```python
from build123d import *

# Parameters (mm, degrees)
F0_W          = 18
F0_H          = 18
F0_W_2        = 10
F0_H_2        = 10
F1_DEPTH      = 4
F2_DEPTH      = 12
F2_TAPER      = 3
F3_SIZE       = 2
F4_R          = 2
F5_W          = 5
F5_H          = 5
F6_DEPTH      = 5
F6_TAPER      = 3
F7_W          = 6
F7_H          = 3
F8_DEPTH      = 25
F8_DEPTH_BACK = 25


with BuildPart() as f1:
    # F0 (on Top) → F1 (new body)
    with BuildSketch(Plane.XY):
        Rectangle(F0_W, F0_H)
        Rectangle(F0_W_2, F0_H_2, mode=Mode.SUBTRACT)
        Rectangle(F0_W_2, F0_H_2)
    extrude(amount=F1_DEPTH)

    # F0 (on Top) → F2 (join)
    with BuildSketch(Plane.XY):
        Rectangle(F0_W_2, F0_H_2)
    extrude(amount=F2_DEPTH, taper=F2_TAPER)

    # F3
    f3_edges = [f1.edges().sort_by_distance(p)[0] for p in [
        (-9, 0, 4),
        (0, -9, 4),
        (9, 0, 4),
        (0, 9, 4),
    ]]
    chamfer(f3_edges, length=F3_SIZE)

    # F4
    f4_edges = [f1.edges().sort_by_distance(p)[0] for p in [
        (0, -4.790369, 4),
        (-4.790369, 0, 4),
        (4.790369, 0, 4),
        (0, 4.790369, 4),
    ]]
    fillet(f4_edges, radius=F4_R)

    # F5 (on face) → F6 (cut)
    with BuildSketch(Plane.XY.offset(12)):
        Rectangle(F5_W, F5_H)
    extrude(amount=-F6_DEPTH, taper=F6_TAPER, mode=Mode.SUBTRACT)

    # F7 (on Front) → F8 (cut, two sides)
    with BuildSketch(Plane.XZ) as f8_sk:
        with Locations((0, 9)):
            Rectangle(F7_W, F7_H)
    extrude(amount=F8_DEPTH, mode=Mode.SUBTRACT)
    extrude(f8_sk.sketch, amount=-F8_DEPTH_BACK, mode=Mode.SUBTRACT)


solid = f1.part
```
Build history of the part. All positions in model axes, mm. A direction names the side the tool comes from. Round coordinates to 2 decimals unless told otherwise and drop trailing zeros. Loops run counter-clockwise (first coordinate to the right, second up) from the corner with the lowest first, then second, coordinate; pieces in that order, holes last. Notation, with made-up numbers: M -14,67.25 L 17,67.25 A20 cw 17,84.25 Z; hole C 31.5,67.5 d2. An arc over 180 degrees is marked long. Answer as CSV lines item,"result".
1. 3-axis set-ups, long thin cutter, end or side, ignore diameter. For faces 5 (the flat face through (0, 0, 7)), 6 (the flat face through (2.6, 0.1, 7.5)), 7 (the flat face through (0, 0, 0)): which of +Z, -Z, +X, -X, +Y, -Y reach the whole face in a straight line?
Resolved:
face 5,"+Z"
face 6,"+Y, -Y"
face 7,"-Z, +X, -X, +Y, -Y"
2. Two-plate mould, pull along Z, no slides. Class faces 1 (the flat face through (-9, 0, 1)), 2 (the flat face through (0, -8, 3)), 3 (the flat face through (3, 0, 9)), 4 (the flat face through (-3, 0, 9)): released by +Z, released by -Z, zero draft, split by the parting line, or undercut.
Resolved:
face 1,"zero draft"
face 2,"released by +Z"
face 3,"undercut"
face 4,"undercut"
3. Wall check: probe 1 along Z at (x, y) = (2.5, -3); probe 2 along X at (y, z) = (-2.25, 9); probe 3 along Z at (x, y) = (-8, 0.5). Give the ranges that are in metal, low to high. Write a range as [from, to].
Resolved:
probe 1,"z = [0, 7.5], [10.5, 12]"
probe 2,"x = [-4.53, -3], [3, 4.53]"
probe 3,"z = [0, 3]"
4. Cut at A-A on x = 2.75. Write the cut outline in (y, z).
Resolved:
outline,"M -9,0 L 9,0 L 9,2 L 7,4 L 6.69,4 A2 cw 4.69,5.9 L 4.61,7.5 L -4.61,7.5 L -4.69,5.9 A2 cw -6.69,4 L -7,4 L -9,2 Z; M -4.45,10.5 L 4.45,10.5 L 4.37,12 L -4.37,12 Z"
5. Cut at B-B on z = 9. Write the cut outline in (x, y).
Resolved:
outline,"M -4.53,-4.53 L -3,-4.53 L -3,4.53 L -4.53,4.53 Z; M 3,-4.53 L 4.53,-4.53 L 4.53,4.53 L 3,4.53 Z"
6. Cut at C-C on y = -4. Write the cut outline in (x, z), then the cut area to 3 significant figures.
Resolved:
outline,"M -9,0 L 9,0 L 9,2 L 7,4 L 6.69,4 A2 cw 4.69,5.9 L 4.37,12 L -4.37,12 L -4.69,5.9 A2 cw -6.69,4 L -7,4 L -9,2 Z; hole M -3,7.5 L 3,7.5 L 3,10.5 L -3,10.5 Z"
area,"125 mm²"
7. Flat gauge pins, fed straight in: P1, Ø5, axis at x = 4, z = 5, coming from the -Y side; P2, Ø1, axis at y = -5, z = 3.5, coming from the -X side; P3, Ø2.5, axis at y = -1.5, z = 9, coming from the +X side. Where does each tip first touch, or does it go through?
Resolved:
P1,"stops at y = -8.5"
P2,"stops at x = -8"
P3,"stops at x = 4.59"
8. Cut at D-D on x = 0.5. Count the separate pieces of the cut face and the enclosed holes in it, then the cut area to 3 significant figures.
Resolved:
separate pieces,"3"
enclosed holes,"0"
area,"106 mm²"
